CAD build for the part. Positions are in the model's coordinates, mm. A direction names the side the tool comes from. Round coordinates to 2 decimals unless told otherwise and drop trailing zeros. Loops run counter-clockwise (first coordinate to the right, second up) from the corner with the lowest first, then second, coordinate; pieces in that order, holes last. Notation, with made-up numbers: M 8,-20.5 L 48,-20.5 A5 cw 48,-11.5 Z; hole C 36.5,19 d1. An arc over 180 degrees is marked long. Put each result on its own line as item: value. Start each with the question number.
Autodesk Inventor part; units mm, degrees
ref_plane "Work Plane1" through (0, 170, 0) normal (0, 1, 0) x (1, 0, 0)
ref_plane "YZ Plane" through (0, 0, 0) normal (1, 0, 0) x (0, 1, 0)
ref_plane "XZ Plane" through (0, 0, 0) normal (0, 1, 0) x (-1, 0, 0)
sketch "Sketch1" plane through (0, 0, 0) normal (0, 1, 0) x (-1, 0, 0)
  circle A0 centre (0, 0) radius 105
  dimension "d0" = 210
extrude "Extrusion1" add sketch "Sketch1" along normal blind 190
sketch "Sketch2" plane through (0, 190, 0) normal (0, 1, 0) x (1, 0, 0)
  circle A0 centre (0, 0) radius 95
  dimension "d3" = 190
extrude "Extrusion2" cut sketch "Sketch2" against normal blind 170
ref_plane "Work Plane1" through (0, 170, 0) normal (0, 1, 0) x (1, 0, 0)
sketch "Sketch3" plane through (0, 170, 0) normal (0, 1, 0) x (1, 0, 0)
  circle A0 centre (0, 0) radius 95
  line L0 (0, 0) -> (20.2008, 0) construction
  line L1 (0, 0) -> (20.2008, 0) construction
  circle A1 centre (0, 0) radius 105
  line L2 (0, 0) -> (10.5, 0) construction
  line L3 (5.449, 7.7819) -> (60.2255, 86.011)
  line L4 (0, 0) -> (10.5, 0) construction
  line L5 (7.7819, 5.449) -> (86.011, 60.2255)
  line L6 (0, 0) -> (10.5, 0) construction
  line L7 (5.449, -7.7819) -> (60.2255, -86.011)
  line L8 (0, 0) -> (10.5, 0) construction
  line L9 (7.7819, -5.449) -> (86.011, -60.2255)
  line L10 (0, 0) -> (10.5, 0) construction
  line L11 (-5.449, 7.7819) -> (-60.2255, 86.011)
  line L12 (0, 0) -> (10.5, 0) construction
  line L13 (-7.7819, 5.449) -> (-86.011, 60.2255)
  line L14 (0, 0) -> (10.5, 0) construction
  line L15 (0, 0) -> (10.5, 0) construction
  line L16 (0, 0) -> (10.5, 0) construction
  line L17 (-5.449, -7.7819) -> (-60.2255, -86.011)
  line L18 (-7.7819, -5.449) -> (-86.011, -60.2255)
  arc A2 (7.7819, 5.449) -> (5.449, 7.7819) centre (0, 0) ccw
  arc A3 (5.449, -7.7819) -> (7.7819, -5.449) centre (0, 0) ccw
  arc A4 (-5.449, 7.7819) -> (-7.7819, 5.449) centre (0, 0) ccw
  arc A5 (-7.7819, -5.449) -> (-5.449, -7.7819) centre (0, 0) ccw
  arc A6 (-60.2255, 86.011) -> (-86.011, 60.2255) centre (0, 0) ccw
  arc A7 (86.011, 60.2255) -> (60.2255, 86.011) centre (0, 0) ccw
  arc A8 (-86.011, -60.2255) -> (-60.2255, -86.011) centre (0, 0) ccw
  arc A9 (60.2255, -86.011) -> (86.011, -60.2255) centre (0, 0) ccw
  point P0 (-77.8194, 54.4898)
  point P1 (-54.4898, 77.8194)
  point P2 (77.8194, -54.4898)
  point P3 (54.4898, -77.8194)
  point P4 (77.8194, 54.4898)
  point P5 (54.4898, 77.8194)
  point P6 (-77.8194, -54.4898)
  point P7 (-54.4898, -77.8194)
  dimension "d22" = 55
  dimension "d23" = 35
  dimension "d24" = 55
  dimension "d26" = 125
  dimension "d27" = 145
extrude "Extrusion3" cut sketch "Sketch3" against normal blind 20 contours A0 L3 A1 L5 | L9 A1 L7 A0 | A0 L13 A1 L11 | L17 A1 L18 A0
(1) Cut at A-A on x = 0. List the corners of the cut face in (y, z).
(2) Drill centre lines: line 1 along Z through (x, y) = (0, 87.5); line 2 along Z through (x, y) = (54, 138); line 3 along Y through (x, z) = (36, -16.5). Where is each one in solid material? Low to high.
(3) Cut at B-B on z = 0. List the corners of the cut face in (x, y), and give its area (3 significant figures).
(4) Flat gauge pins, fed straight in: pin 1 Ø8 at (y, z) = (163.5, 50.5) entering from +X; pin 2 Ø1 at (y, z) = (151.5, 8) entering from -X; pin 3 Ø4 at (y, z) = (109, -42) entering from +X. Where does each tip first touch, or does it go through?
(5) Cut at D-D on y = 12.5. List the corners of the cut face in (x, z).
(6) Tool access for faces 4 (the flat face through (57.32, 160.14, -81.86)), 5 (the cylindrical face through (90.61, 106.19, -28.54)), 6 (the flat face through (-81.86, 160.14, 57.32)), 7 (the cylindrical face through (-100.15, 93.67, -31.54)), 8 (the flat face through (-81.86, 160.14, -57.32)): list every direction of +Z, -Z, +X, -X, +Y, -Y with a clear straight run to the whole face (end or side of a thin tool).
(7) Mould opens along X. For faces 1 (the flat face through (-1, 20, -1)), 2 (the flat face through (57.32, 160.14, 81.86)), 3 (the flat face through (-57.32, 160.14, 81.86)) say: +X half, -X half, draft (parallel to the pull), parting line (faces both ways), or undercut.
(8) Cut at C-C on y = 59. List the corners of the cut face in (x, z), and give its area (3 significant figures).
Taken from the geometry:
1. outline: M 0,-105 L 190,-105 L 190,-95 L 20,-95 L 20,95 L 190,95 L 190,105 L 0,105 Z
2. line 1: -105 to -95, 95 to 105
2. line 2: -90.05 to -78.16, 78.16 to 90.05
2. line 3: 0 to 20
3. outline: M -105,0 L 105,0 L 105,190 L 95,190 L 95,20 L -95,20 L -95,190 L -105,190 Z
3. area: 7,600 mm2
4. pin 1: x = 94.14
4. pin 2: x = -104.73
4. pin 3: x = 97.08
5. outline: C 0,0 d210
6. face 4: +X
6. face 5: +Y
6. face 6: +Z
6. face 7: +Y, -Y
6. face 8: -Z
7. face 1: undercut
7. face 2: +X half
7. face 3: -X half
8. outline: C 0,0 d210; hole C 0,0 d190
8. area: 6,280 mm2
